The figure shows three views and two pictorial views of one solid part (mm, origin at its lowest corner). Answer the questions. A direction names the side the tool comes from. Coordinates: 2 decimals unless noted, no trailing zeros. Order: outer loops, then holes, each group sorted by start corner. A loop starts at its lowest first (then second) coordinate and runs counter-clockwise, first axis right, second up. Notation, with made-up numbers: (-10, 6.25) - (30, 6.25) arc R27 ccw to (30, 28.25) - close; hole circle Ø7 at (-23.5, -3). An arc over 180 degrees is marked (long way). Use one line per item in the form item = value.
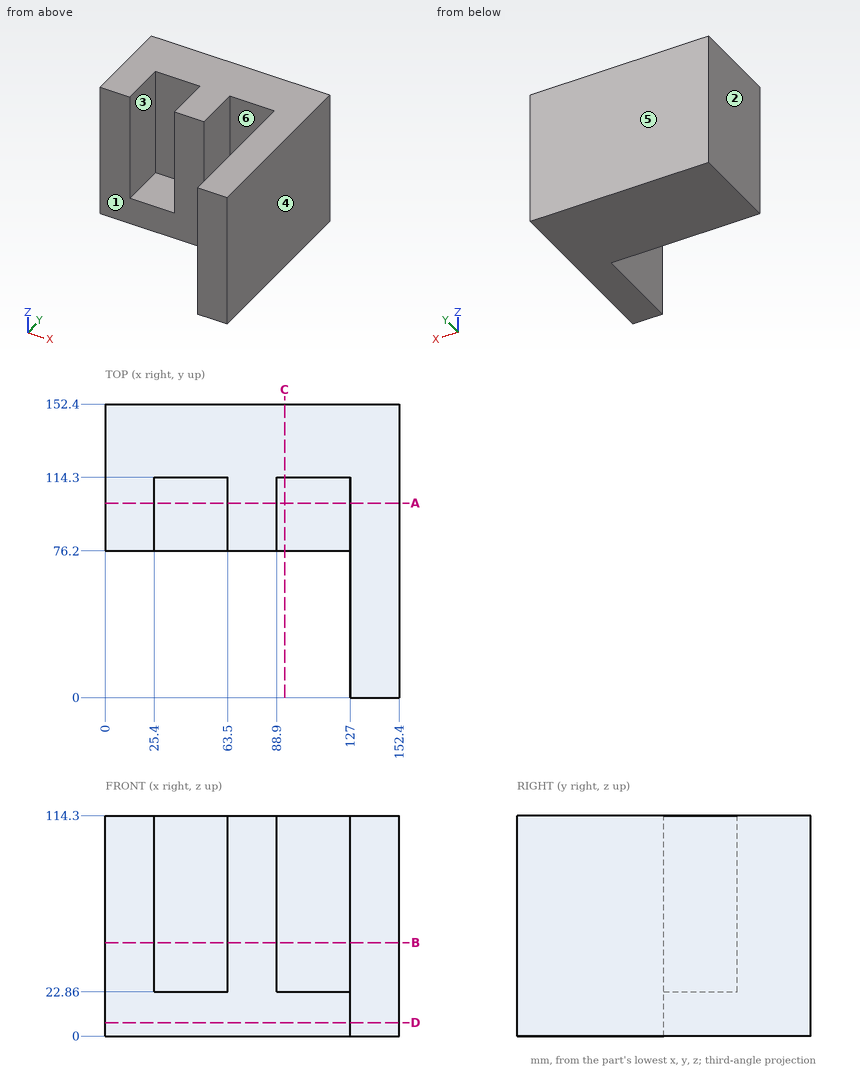
(1) Given pin 1 Ø11.5 at (x, z) = (117, 73.5) entering from -Y; pin 2 Ø11.5 at (x, y) = (105.5, 99) entering from +Z; pin 3 Ø10 at (x, z) = (66, 94) entering from -Y, each flat-ended and moving along its own axis, determine where each tip first touches the part or whether it passes through.
Answer list:
pin_1 = 114.3
pin_2 = 22.86
pin_3 = 76.2
(2) Section D-D, the plane z = 7 is taken. Write down the section's boundary in (x, y).
Answer list:
outline = (0, 76.2) - (127, 76.2) - (127, 0) - (152.4, 0) - (152.4, 152.4) - (0, 152.4) - close
(3) Section A-A, the plane y = 101 is taken. Write down the section's boundary in (x, z).
Answer list:
outline = (0, 0) - (152.4, 0) - (152.4, 114.3) - (127, 114.3) - (127, 22.86) - (88.9, 22.86) - (88.9, 114.3) - (63.5, 114.3) - (63.5, 22.86) - (25.4, 22.86) - (25.4, 114.3) - (0, 114.3) - close
(4) Which of the six approach directions +Z, -Z, +X, -X, +Y, -Y give full straight-line access (tool end or side, diameter ignored) to the marked faces 1, 2 and 3?
Answer list:
face_1 = +Z, -Z, -X, -Y
face_2 = +Z, -Z, -X, +Y, -Y
face_3 = +Z, -Y
(5) Section B-B, the plane z = 48.5 is taken. Write down the section's boundary in (x, y).
Answer list:
outline = (0, 76.2) - (25.4, 76.2) - (25.4, 114.3) - (63.5, 114.3) - (63.5, 76.2) - (88.9, 76.2) - (88.9, 114.3) - (127, 114.3) - (127, 0) - (152.4, 0) - (152.4, 152.4) - (0, 152.4) - close
(6) The mould has two halves that part along X. Classify the marked faces 4, 5 and 6: +X half, -X half, draft (parallel to the pull), parting line (faces both ways), or undercut.
Answer list:
face_4 = +X half
face_5 = draft
face_6 = undercut
(7) Section C-C, the plane x = 93 is taken. Write down the section's boundary in (y, z), then the cut area to 3 significant figures.
Answer list:
outline = (76.2, 0) - (152.4, 0) - (152.4, 114.3) - (114.3, 114.3) - (114.3, 22.86) - (76.2, 22.86) - close
area = 5,230 mm2
(8) Straight lines are drawn through the part: L1, parallel to X at y = 101.5, z = 102; L2, parallel to Y at x = 56, z = 6; L3, parallel to Z at x = 122, y = 97.5. For each, find the intervals that lie inside material, in ascending order.
Answer list:
L1 = 0 to 25.4, 63.5 to 88.9, 127 to 152.4
L2 = 76.2 to 152.4
L3 = 0 to 22.86
